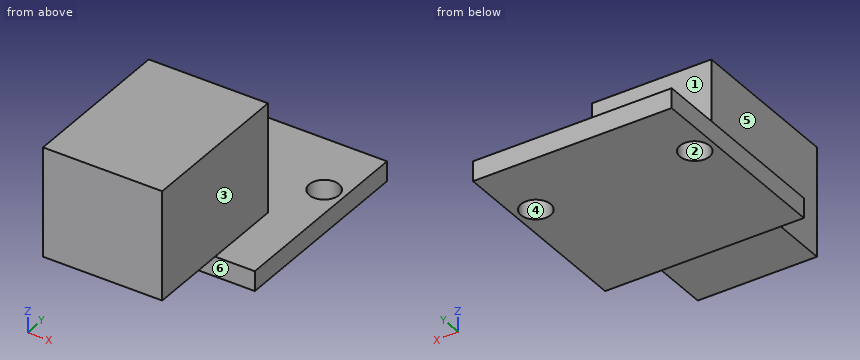
Autodesk Fusion 360 part; units mm, degrees
sketch "Sketch1" plane through (0, 0, 0) normal (0, 0, 1) x (1, 0, 0)
  line L0 (0, 0) -> (20, 0)
  line L1 (20, 0) -> (20, 20)
  line L2 (20, 20) -> (0, 20)
  line L3 (0, 20) -> (0, 0)
  line L4 (4, 8) -> (16, 8)
  line L5 (16, 8) -> (16, -8)
  line L6 (16, -8) -> (4, -8)
  line L7 (4, -8) -> (4, 8)
  line L8 (4, 8) -> (16, -8) construction
  line L9 (16, 8) -> (4, -8) construction
  line L10 (20, 20) -> (0, 20)
  line L11 (0, 20) -> (0, 13.5)
  line L12 (0, 13.5) -> (20, 13.5)
  line L13 (20, 13.5) -> (20, 20)
  line L14 (0, 20) -> (2, 20)
  line L15 (2, 20) -> (2, 13.5)
  line L16 (2, 13.5) -> (0, 13.5)
  line L17 (0, 13.5) -> (0, 20)
  line L18 (20, 20) -> (18, 20)
  line L19 (18, 20) -> (18, 13.5)
  line L20 (18, 13.5) -> (20, 13.5)
  line L21 (20, 13.5) -> (20, 20)
  circle A0 centre (2, 13.5) radius 1.5
  circle A1 centre (18, 13.5) radius 1.5
  point P0 (10, 0)
  dimension "d1" = 20
  dimension "d2" = 20
  dimension "d3" = 16
  dimension "d4" = 20
  dimension "d5" = 6.5
  dimension "d6" = 2
  dimension "d7" = 2
extrude "Extrude1" add sketch "Sketch1" against normal blind 2 contours L0 L1 L3 L4 L5 L7 L12 L16 L20 A0 A1 | L0 L4 L5 L7 | L2 L3 L10 L11 L12 L14 L15 L16 L17 A0 | L2 L10 L12 L15 L19 A0 A1 | L1 L2 L10 L12 L13 L18 L19 L20 L21 A1
extrude "Extrude2" add sketch "Sketch1" along normal blind 11 contours L0 L4 L5 L7 | L0 L5 L6 L7
For this review, take the finished solid that the model builds, in its own axes (mm). Face numbers are marked on the shaded views. A direction names the side the tool comes from. Coordinates: 2 decimals unless noted, no trailing zeros. Loops run counter-clockwise (first coordinate to the right, second up) from the corner with the lowest first, then second, coordinate; pieces in that order, holes last. Notation, with made-up numbers: (17.25, -22.5) - (36.25, -22.5) arc R13 ccw to (36.25, -6.5) - close; hole circle Ø3 at (65, -2). An arc over 180 degrees is marked (long way). Use one line per item in the form item = value. Start each with the question number.
1) Take a section at A-A (y = 13.5). State the section outline as (x, z) points, plus the area to 3 significant figures.
2) Take a section at B-B (x = 17.75). State the section outline as (y, z) points.
3) For pin 1 (2 mm diameter, centred on x = 13, z = -1.5, fed in from -Y); pin 2 (1 mm diameter, centred on y = -1, z = 9, fed in from +X); pin 3 (5.5 mm diameter, centred on y = -1.5, z = 8, fed in from -X); pin 4 (2.5 mm diameter, centred on x = 2, y = 13.5, fed in from +Z), all flat-tipped, find the tip position at first contact; note any pin that passes through.
4) For the marked faces 4, 5 and 6, list the 3-axis set-ups (+Z, -Z, +X, -X, +Y, -Y) from which the entire face can be reached by the end or side of a thin tool; tool diameter is ignored.
5) Take a section at D-D (x = 11.25). State the section outline as (y, z) points, plus the area to 3 significant figures.
6) Draft analysis for pull direction X (two halves, no side actions). For the marked faces 1, 2 and 3, state which applies: released by +X, released by -X, zero draft, split by the parting line, or undercut.
7) To check wall thickness, follow probe 1 along X at (y, z) = (13.5, -1); probe 2 along Y at (x, z) = (2, -1); probe 3 along Z at (x, y) = (5.75, 15.25). State the ranges of each line that lie inside material, in increasing order. Write a range as from..to.
8) Take a section at C-C (z = -0.75). State the section outline as (x, y) points.
From the geometry:
q1.outline = (0, -2) - (0.5, -2) - (0.5, 0) - (0, 0) - close; (3.5, -2) - (16.5, -2) - (16.5, 0) - (3.5, 0) - close; (19.5, -2) - (20, -2) - (20, 0) - (19.5, 0) - close
q1.area = 28.0 mm2
q2.outline = (0, -2) - (12.02, -2) - (12.02, 0) - (0, 0) - close; (14.98, -2) - (20, -2) - (20, 0) - (14.98, 0) - close
q3.pin_1 = 0
q3.pin_2 = 16
q3.pin_3 = 4
q3.pin_4 = through
q4.face_4 = +Z, -Z
q4.face_5 = +Z, -X, +Y, -Y
q4.face_6 = -Z, +X, -X, -Y
q5.outline = (-8, 0) - (0, 0) - (0, -2) - (20, -2) - (20, 0) - (8, 0) - (8, 11) - (-8, 11) - close
q5.area = 216 mm2
q6.face_1 = zero draft
q6.face_2 = undercut
q6.face_3 = released by +X
q7.probe_1 = 0..0.5, 3.5..16.5, 19.5..20
q7.probe_2 = 0..12, 15..20
q7.probe_3 = -2..0
q8.outline = (0, 0) - (20, 0) - (20, 20) - (0, 20) - close; hole circle Ø3 at (2, 13.5); hole circle Ø3 at (18, 13.5)
